Source: three-view drawing plus pictorial views. Frame: mm from the lowest corner of the part. A direction names the side the tool comes from. Give positions to 0.01 mm unless a question says otherwise; leave off trailing zeros. Loops run counter-clockwise (first coordinate to the right, second up) from the corner with the lowest first, then second, coordinate; pieces in that order, holes last. Notation, with made-up numbers: (34, 67) - (66, 67) arc R20 ccw to (66, 88) - close; hole circle Ø6 at (30, 88.25). An arc over 180 degrees is marked (long way). One line per item, written item: value.
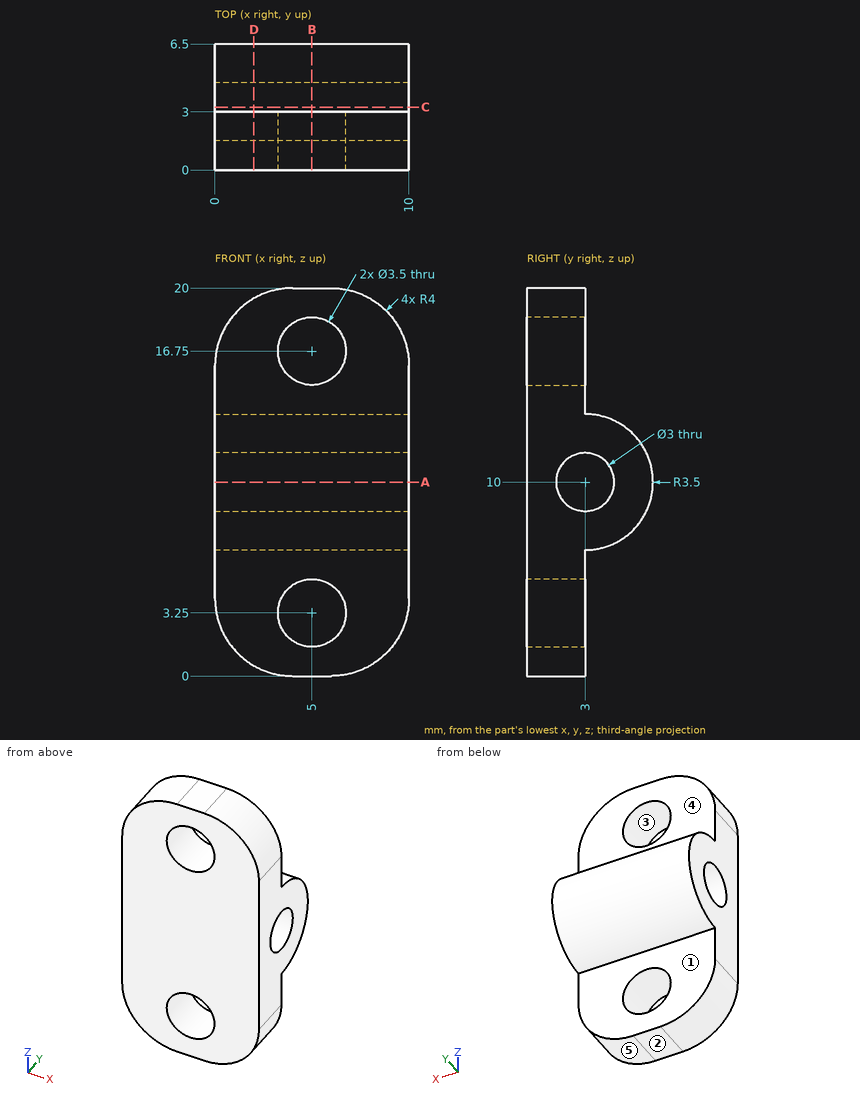
Item 1: Section C-C, the plane y = 3.25. Output: boundary loops of the cut face in (x, z).
Verdict:
outline: (0, 6.51) - (10, 6.51) - (10, 8.52) - (0, 8.52) - close; (0, 11.48) - (10, 11.48) - (10, 13.49) - (0, 13.49) - close
Item 2: Section D-D, the plane x = 2. Output: boundary loops of the cut face in (y, z).
Verdict:
outline: (0, 0.54) - (3, 0.54) - (3, 6.5) arc R3.5 ccw to (3, 13.5) - (3, 19.46) - (0, 19.46) - close; hole circle Ø3 at (3, 10)
Item 3: Pin query (flat end, axial travel): P1, Ø2, axis at x = 3.5, z = 11.5, coming from the +Y side; P2, Ø2.5, axis at y = 3, z = 10, coming from the -X side; P3, Ø2, axis at x = 2.5, z = 17, coming from the +Y side. Return the tip coordinate at first contact, or that it passes through.
Verdict:
P1: stops at y = 6.46
P2: passes through
P3: stops at y = 3
Item 4: Access query for the marked faces 1 and 2. Directions: +Z, -Z, +X, -X, +Y, -Y. A direction counts if a zero-diameter tool reaches every point of the face in a straight line with its end or side. Return the directions, or none.
Verdict:
face 1: -Z, +X, -X, +Y
face 2: -Z, +X, -X, +Y, -Y
Item 5: Material intervals for L1, parallel to Y at x = 7, z = 10; L2, parallel to Y at x = 4.25, z = 14; L3, parallel to Z at x = 4.5, y = 1, sorted ascending.
Verdict:
L1: y = 0 to 1.5, 4.5 to 6.5
L2: y = 0 to 3
L3: z = 0 to 1.57, 4.93 to 15.07, 18.43 to 20
Item 6: Section A-A, the plane z = 10. Output: boundary loops of the cut face in (x, y), and give its area (3 significant figures).
Verdict:
outline: (0, 0) - (10, 0) - (10, 1.5) - (0, 1.5) - close; (0, 4.5) - (10, 4.5) - (10, 6.5) - (0, 6.5) - close
area: 35.0 mm^2
Item 7: Section B-B, the plane x = 5. Output: boundary loops of the cut face in (y, z), and give its area (3 significant figures).
Verdict:
outline: (0, 0) - (3, 0) - (3, 1.5) - (0, 1.5) - close; (0, 5) - (3, 5) - (3, 6.5) arc R3.5 ccw to (3, 13.5) - (3, 15) - (0, 15) - close; (0, 18.5) - (3, 18.5) - (3, 20) - (0, 20) - close; hole circle Ø3 at (3, 10)
area: 51.2 mm^2
Item 8: Draft query along X for the marked faces 3, 4 and 5. Return one class per face: pulls with the +X half, pulls with the -X half, needs draft (parallel to the pull), parting line crosses it, or undercut.
Verdict:
face 3: undercut
face 4: needs draft
face 5: pulls with the +X half
